Job drawing, mm, ordinate dimensions from the low corner. One solid piece. A direction names the side the tool comes from. Coordinates: 2 decimals unless noted, no trailing zeros. Write each loop counter-clockwise with the first axis right and the second up, starting at its lowest first coordinate (ties: lowest second). Pieces come first, ordered by that corner, then holes. Notation, with made-up numbers: (76, 51) - (90, 51) arc R18 cw to (90, 81) - close; hole circle Ø2 at (-24.5, -34). An arc over 180 degrees is marked (long way). Use a Markdown table: item, result.
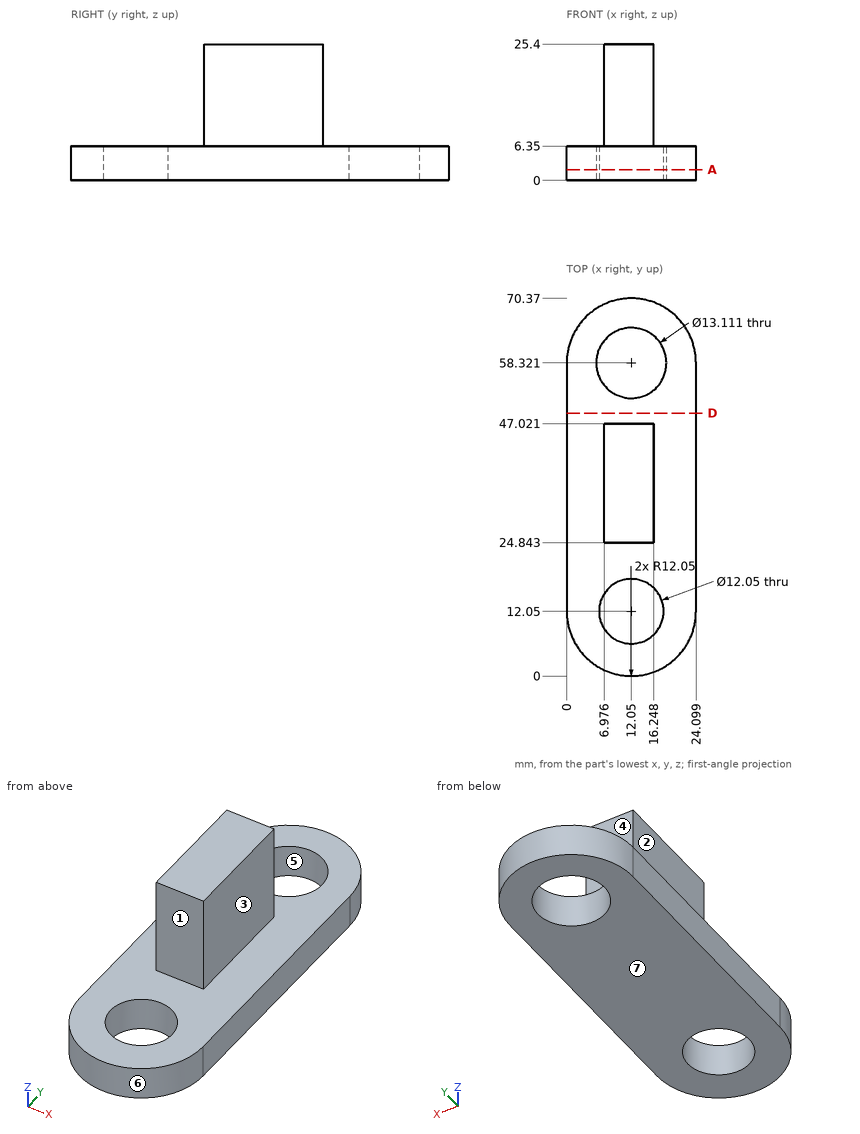
Item 1: Which spindle directions (+Z, -Z, +X, -X, +Y, -Y) get a long thin tool onto all of the face, cutting with end or side? Do the marked faces 1, 2, 3 and 4. Say none if no direction does.
From the geometry:
| item | result |
|---|---|
| face 1 | +Z, +X, -X, -Y |
| face 2 | +Z, -X, +Y, -Y |
| face 3 | +Z, +X, +Y, -Y |
| face 4 | +Z, +X, -X, +Y |
Item 2: Band-saw the part on A-A, the plane z = 2. Count the separate pieces of the cut face and the enclosed holes in it, then the cut area to 3 significant figures.
From the geometry:
| item | result |
|---|---|
| separate pieces | 1 |
| enclosed holes | 2 |
| area | 1,320 mm^2 |
Item 3: Two-plate mould, pull along Y, no slides. Class the marked faces 5, 6 and 7: pulls with the +Y half, pulls with the -Y half, needs draft (parallel to the pull), parting line crosses it, or undercut.
From the geometry:
| item | result |
|---|---|
| face 5 | undercut |
| face 6 | pulls with the -Y half |
| face 7 | needs draft |
Item 4: Band-saw the part on D-D, the plane y = 49. Give the cut face in (x, z).
From the geometry:
| item | result |
|---|---|
| outline | (0, 0) - (24.1, 0) - (24.1, 6.35) - (0, 6.35) - close |
Item 5: Drop flat-ended pins along their axis: P1, Ø15, axis at y = 32, z = 14, coming from the +X side; P2, Ø4.5, axis at x = 12.5, z = 11.5, coming from the +Y side; P3, Ø5, axis at x = 17.5, y = 52, coming from the +Z side; P4, Ø9.5, axis at x = 12.05, y = 12.05, coming from the +Z side. Give the stop position or say it passes through.
From the geometry:
| item | result |
|---|---|
| P1 | x = 16.25 |
| P2 | y = 47.02 |
| P3 | z = 6.35 |
| P4 | through |
Item 6: Drill centre lines: probe 1 along Y at (x, z) = (15.25, 4.5) (1 decimal); probe 2 along Z at (x, y) = (6, 53); probe 3 along Y at (x, z) = (14.5, 12.75). Where is each one in solid material? Low to high.
From the geometry:
| item | result |
|---|---|
| probe 1 | 0.4 to 6.9, 17.2 to 52.6, 64 to 69.9 |
| probe 2 | 0 to 6.35 |
| probe 3 | 24.84 to 47.02 |
